Geometry check sheet. Reference: the model listing, model coordinates, mm. A direction names the side the tool comes from. Give positions to 0.01 mm unless a question says otherwise; leave off trailing zeros. Loops run counter-clockwise (first coordinate to the right, second up) from the corner with the lowest first, then second, coordinate; pieces in that order, holes last. Notation, with made-up numbers: (56.5, -5.5) - (94.5, -5.5) arc R18 cw to (94.5, 18.5) - close; hole circle Ø4 at (69.5, 53). An arc over 180 degrees is marked (long way). One line per question, with ' | ' between items. Start each with the question number.
Autodesk Inventor part; units mm, degrees
ref_plane "YZ Plane" through (0, 0, 0) normal (1, 0, 0) x (0, 1, 0)
ref_plane "XZ Plane" through (0, 0, 0) normal (0, 1, 0) x (-1, 0, 0)
ref_plane "XY Plane" through (0, 0, 0) normal (0, 0, 1) x (1, 0, 0)
sketch "Sketch1" plane through (0, 0, 0) normal (0, 1, 0) x (-1, 0, 0)
  circle A0 centre (0, 0) radius 5
  arc A1 (-5.8378, -12.1725) -> (-5.8378, 12.1725) centre (0, 0) ccw
  circle A2 centre (18.5, 0) radius 2.5
  circle A3 centre (-18.5, 0) radius 2.5
  line L0 (0, -18.9) -> (0, 18.9)
  line L1 (20.8784, 4.9592) -> (5.8378, 12.1725)
  line L2 (33.6, 0) -> (-33.6, 0)
  line L3 (20.8784, -4.9592) -> (5.8378, -12.1725)
  line L4 (-20.8784, 4.9592) -> (-5.8378, 12.1725)
  line L5 (-20.8784, -4.9592) -> (-5.8378, -12.1725)
  arc A4 (-20.8784, 4.9592) -> (-20.8784, -4.9592) centre (-18.5, 0) ccw
  arc A5 (20.8784, -4.9592) -> (20.8784, 4.9592) centre (18.5, 0) ccw
  dimension "d0" = 10
  dimension "d1" = 27
  dimension "d2" = 5
  dimension "d3" = 5
  dimension "d4" = 37
  dimension "d5" = 18.5
extrude "Extrusion1" add sketch "Sketch1" along normal blind 4 contours L2 A1 L0 A0 | A0 L0 A1 L2 | A0 L2 A3 A4 L4 A1 L0 | L0 A1 L5 A4 L2 A3 A0 | L2 A2 A5 L3 A1 | A1 L1 A5 L2 A2
sketch "Sketch2" plane through (0, 0, 0) normal (0, -1, 0) x (1, 0, 0)
  circle A0 centre (0, 0) radius 5
  circle A1 centre (0, 0) radius 13
  dimension "d11" = 26
  dimension "d23" = 10
extrude "Extrusion2" add sketch "Sketch2" along normal blind 4.5
sketch "Sketch3" plane through (0, -4.5, 0) normal (0, -1, 0) x (1, 0, 0)
  circle A0 centre (0, 0) radius 5
  circle A1 centre (0, 0) radius 5
  circle A2 centre (0, 0) radius 7.5
  dimension "d14" = 15
  dimension "d24" = 10
extrude "Extrusion3" add sketch "Sketch3" along normal blind 3.5
sketch "Sketch4" plane through (0, -4.5, 0) normal (0, -1, 0) x (1, 0, 0)
  circle A0 centre (0, 0) radius 5.5
  circle A1 centre (0, 0) radius 7.5
  circle A2 centre (0, 0) radius 11
  dimension "d17" = 22
extrude "Extrusion4" cut sketch "Sketch4" against normal blind 0.5 contours A1 | A2
sketch "Sketch5" plane through (0, -4, 0) normal (0, -1, 0) x (1, 0, 0)
  circle A0 centre (0, 0) radius 5.5
  circle A1 centre (0, 0) radius 10.5
  dimension "d20" = 21
extrude "Extrusion5" cut sketch "Sketch5" against normal blind 0.2
properties part number "Kep Truc KLF-08"
(1) Mould release check, pull along Z, two halves, no side actions. Record for faces 4 (the face through (2, -8, -5)), 5 (the face through (-2.38, -4.25, -10.74)), 6 (the face through (-10.316, -2.218, 7.91)): pulls with the +Z half, pulls with the -Z half, needs draft (parallel to the pull), parting line crosses it, or undercut.
(2) Section check A-A, the plane y = 2.75. Record the boundary of the cut face in (x, z).
(3) Section check D-D, the plane y = -1.25. Record the boundary of the cut face in (x, z).
(4) Tool access check on faces 1 (the face through (-1.19, -4.15, -5.37)), 2 (the face through (-11, -4.5, 3)), 3 (the face through (6, 4, 0)). Record the directions out of +Z, -Z, +X, -X, +Y, -Y that give a thin tool (end or side, any length) a straight path to the whole face; none if there is none.
(5) Material ranges on line 1 (Z direction, x = 0, y = -5.45); line 2 (X direction, y = 0.9, z = 0); line 3 (Y direction, x = 16, z = 2.25), recorded low to high.
(6) Depth check by flat-ended pin: pin 1 Ø6 at (x, y) = (12, -2.5) entering from +Z; pin 2 Ø1 at (y, z) = (-2, 3) entering from -X; pin 3 Ø3 at (x, y) = (-10, -4.5) entering from -Z. Enter the tip coordinate at first touch or a pass-through.
(7) Section check B-B, the plane x = 0. Record the boundary of the cut face in (y, z), and give its area (3 significant figures).
(8) Section check C-C, the plane z = -6.5. Record the boundary of the cut face in (x, y), and give its area (3 significant figures).
Numbers:
1) face 4: needs draft | face 5: undercut | face 6: parting line crosses it
2) outline: (-20.88, -4.96) - (-5.84, -12.17) arc R13.5 ccw to (5.84, -12.17) - (20.88, -4.96) arc R5.5 ccw to (20.88, 4.96) - (5.84, 12.17) arc R13.5 ccw to (-5.84, 12.17) - (-20.88, 4.96) arc R5.5 ccw to start; hole circle Ø5 at (-18.5, 0); hole circle Ø10 at (0, 0); hole circle Ø5 at (18.5, 0)
3) outline: circle Ø26 at (0, 0); hole circle Ø10 at (0, 0)
4) face 1: none | face 2: -Y | face 3: +Z, -Z, +X, -X, +Y
5) line 1: -7.5 to -5, 5 to 7.5 | line 2: -24 to -21, -16 to -5, 5 to 16, 21 to 24 | line 3: 0 to 4
6) pin 1: z = 10.01 | pin 2: x = -12.76 | pin 3: z = -9.84
7) outline: (-8, -7.5) - (-4.5, -7.5) - (-4.5, -5.5) - (-3.8, -5.5) - (-3.8, -10.5) - (-4, -10.5) - (-4, -11) - (-4.5, -11) - (-4.5, -13) - (0, -13) - (0, -13.5) - (4, -13.5) - (4, -5) - (-8, -5) - close; (-8, 5) - (4, 5) - (4, 13.5) - (0, 13.5) - (0, 13) - (-4.5, 13) - (-4.5, 11) - (-4, 11) - (-4, 10.5) - (-3.8, 10.5) - (-3.8, 5.5) - (-4.5, 5.5) - (-4.5, 7.5) - (-8, 7.5) - close | area: 150 mm^2
8) outline: (-17.67, 0) - (-11.26, 0) - (-11.26, -4.5) - (-8.87, -4.5) - (-8.87, -4) - (-8.25, -4) - (-8.25, -3.8) - (8.25, -3.8) - (8.25, -4) - (8.87, -4) - (8.87, -4.5) - (11.26, -4.5) - (11.26, 0) - (17.67, 0) - (17.67, 4) - (-17.67, 4) - close; (-3.74, -8) - (3.74, -8) - (3.74, -4.5) - (-3.74, -4.5) - close | area: 257 mm^2
